Verification items for this drawing (mm, ordinates from the low corner). A direction names the side the tool comes from. Coordinates: 2 decimals unless noted, no trailing zeros. Write each loop counter-clockwise with the first axis right and the second up, starting at its lowest first coordinate (ties: lowest second). Pieces come first, ordered by that corner, then holes. Notation, with made-up numbers: (7.25, -1.75) -> (19.25, -1.75) arc R10 ccw to (19.25, 13.25) -> close; hole circle Ø6 at (-33, 86). An arc over 180 degrees is marked (long way). One line per question, with ' | ' between items.
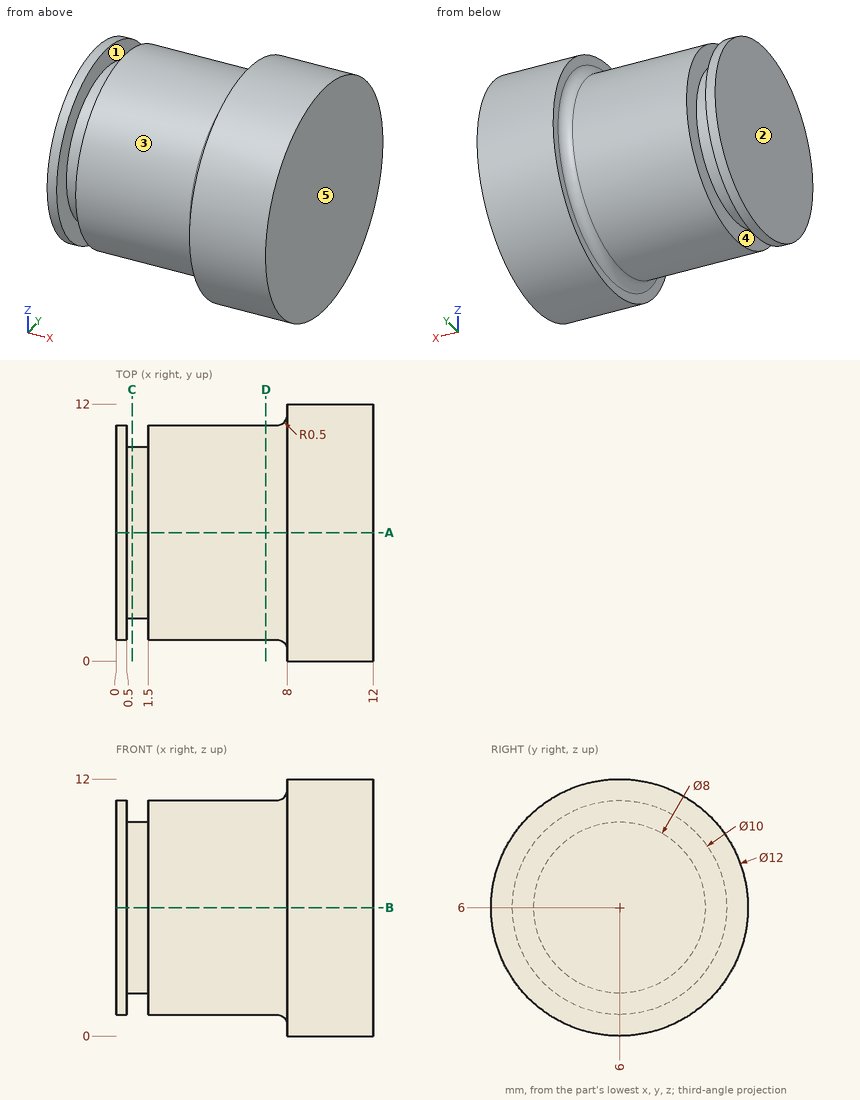
(1) Tool access check on the marked faces 4 and 5. Record the directions out of +Z, -Z, +X, -X, +Y, -Y that give a thin tool (end or side, any length) a straight path to the whole face; none if there is none.
Answers below:
face 4: none | face 5: +Z, -Z, +X, +Y, -Y
(2) Material ranges on line 1 (X direction, y = 5.75, z = 1.75); line 2 (X direction, y = 11.5, z = 5); line 3 (Y direction, x = 8.25, z = 3.5), recorded low to high.
Answers below:
line 1: x = 0 to 0.5, 1.5 to 12 | line 2: x = 8 to 12 | line 3: y = 0.55 to 11.45
(3) Cross-section at D-D (x = 7). Record the cut outline in (y, z), plus the area to 3 significant figures.
Answers below:
outline: circle Ø10 at (6, 6) | area: 78.5 mm²
(4) Cross-section at C-C (x = 0.75). Record the cut outline in (y, z), plus the area to 3 significant figures.
Answers below:
outline: circle Ø8 at (6, 6) | area: 50.3 mm²
(5) Draft check along X on the marked faces 1, 2 and 3. Enter one of: pulls with the +X half, pulls with the -X half, needs draft (parallel to the pull), parting line crosses it, or undercut.
Answers below:
face 1: undercut | face 2: pulls with the -X half | face 3: needs draft
(6) Cross-section at A-A (y = 6). Record the cut outline in (x, z), plus the area to 3 significant figures.
Answers below:
outline: (0, 1) -> (0.5, 1) -> (0.5, 2) -> (1.5, 2) -> (1.5, 1) -> (7.5, 1) arc R0.5 cw to (8, 0.5) -> (8, 0) -> (12, 0) -> (12, 12) -> (8, 12) -> (8, 11.5) arc R0.5 cw to (7.5, 11) -> (1.5, 11) -> (1.5, 10) -> (0.5, 10) -> (0.5, 11) -> (0, 11) -> close | area: 126 mm²
(7) Depth check by flat-ended pin: P1, Ø6, axis at x = 5, z = 10, coming from the +Y side; P2, Ø1.5, axis at x = 10, z = 8.5, coming from the +Y side; P3, Ø6, axis at x = 9, y = 1.5, coming from the +Z side. Enter the tip coordinate at first touch or a pass-through.
Answers below:
P1: stops at y = 10.9 | P2: stops at y = 11.74 | P3: stops at z = 11.81
